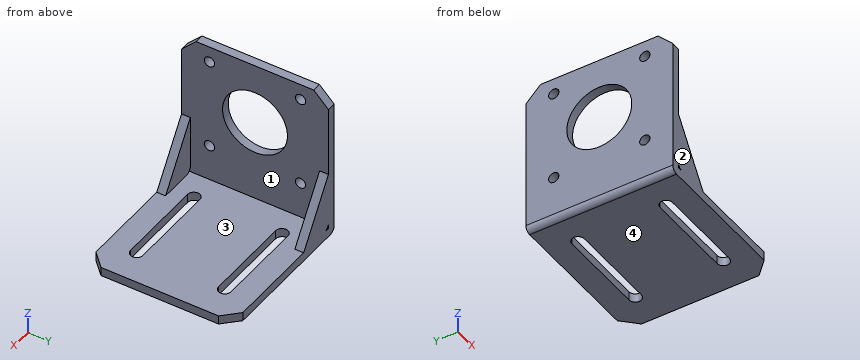
```python
from build123d import *

# Parameters (mm, degrees)
SKETCH_1_W      = 53
SKETCH_1_H      = 50
EXTRUDE_1_DEPTH = 3
SKETCH_2_W      = 49
SKETCH_2_H      = 50
SKETCH_2_R      = 11.05
SKETCH_2_R_2    = 1.75
EXTRUDE_2_DEPTH = 3
CHAMFER_1_SIZE  = 5
EXTRUDE_3_DEPTH = 3
FILLET_1_R      = 2


with BuildPart() as part:
    # 草图1 → 凸台-拉伸1 (new body)
    with BuildSketch(Plane.XY):
        Rectangle(SKETCH_1_W, SKETCH_1_H)
        with BuildLine():
            Line((-14.5, 17.103323548), (15.5, 17.103323548))
            ThreePointArc((15.5, 17.103323548), (17.603323548, 15), (15.5, 12.896676452))
            Line((15.5, 12.896676452), (-14.5, 12.896676452))
            ThreePointArc((-14.5, 12.896676452), (-16.603323548, 15), (-14.5, 17.103323548))
        make_face(mode=Mode.SUBTRACT)
        with BuildLine():
            Line((-14.5, -12.9), (15.5, -12.9))
            ThreePointArc((15.5, -12.9), (17.6, -15), (15.5, -17.1))
            Line((15.5, -17.1), (-14.5, -17.1))
            ThreePointArc((-14.5, -17.1), (-16.6, -15), (-14.5, -12.9))
        make_face(mode=Mode.SUBTRACT)
    extrude(amount=EXTRUDE_1_DEPTH)

    # 草图2 → 凸台-拉伸2 (add)
    with BuildSketch(Plane.ZY.offset(26.5)):
        with Locations((27.5, 0)):
            Rectangle(SKETCH_2_W, SKETCH_2_H)
        with Locations((31, 0)):
            Circle(SKETCH_2_R, mode=Mode.SUBTRACT)
        with Locations((46.5, 15.5)):
            Circle(SKETCH_2_R_2, mode=Mode.SUBTRACT)
        with Locations((46.5, -15.5)):
            Circle(SKETCH_2_R_2, mode=Mode.SUBTRACT)
        with Locations((15.5, -15.5)):
            Circle(SKETCH_2_R_2, mode=Mode.SUBTRACT)
        with Locations((15.5, 15.5)):
            Circle(SKETCH_2_R_2, mode=Mode.SUBTRACT)
    extrude(amount=-EXTRUDE_2_DEPTH)

    # 倒角1
    chamfer_1_edges = [part.edges().sort_by_distance(p)[0] for p in [
        (-25, 25, 52),
        (-25, -25, 52),
        (26.5, 25, 1.5),
        (26.5, -25, 1.5),
    ]]
    chamfer(chamfer_1_edges, length=CHAMFER_1_SIZE)

    # 草图3 → 凸台-拉伸3 (add)
    with BuildSketch(Plane.XZ.offset(25)):
        with BuildLine():
            Line((-23.5, 5), (-23.5, 23))
            Line((-23.5, 23), (-10.5, 3))
            Line((-10.5, 3), (-21.5, 3))
            ThreePointArc((-21.5, 3), (-22.914213562, 3.585786438), (-23.5, 5))
        make_face()
    extrude_3 = extrude(amount=-EXTRUDE_3_DEPTH)

    # 圆角1
    fillet_1_edges = [part.edges().sort_by_distance(p)[0] for p in [
        (-26.5, 0, 0),
    ]]
    fillet(fillet_1_edges, radius=FILLET_1_R)

    # 镜向1: 凸台-拉伸3 across plane
    add(extrude_3.mirror(Plane.ZX))


solid = part.part
```
Read the model definition and answer for the solid it produces. Units are mm, in the model's axes. Face numbers are marked on the shaded views. Give positions to 0.01 mm unless a question says otherwise; leave off trailing zeros. Write each loop counter-clockwise with the first axis right and the second up, starting at its lowest first coordinate (ties: lowest second). Pieces come first, ordered by that corner, then holes. Notation, with made-up numbers: (27.25, 69) -> (35.25, 69) arc R17 cw to (35.25, 81) -> close; hole circle Ø2 at (87, 29). An arc over 180 degrees is marked (long way). Answer as a JSON object with one key per item and string values.
1) Straight lines are drawn through the part: probe 1 along Y at (x, z) = (-24.8, 46.5); probe 2 along Y at (x, z) = (-24.75, 31); probe 3 along Z at (x, y) = (21, -21). For each, find the intervals that lie inside material, in ascending order. Write a range as from..to.
Findings below:
{"probe 1": "y = -25..-17.25, -13.75..13.75, 17.25..25", "probe 2": "y = -25..-11.05, 11.05..25", "probe 3": "z = 0..3"}
2) For a pull along Y with two mould halves and no side action, classify the marked faces 1, 2, 3 and 4 as pulls with the +Y half, pulls with the -Y half, needs draft (parallel to the pull), parting line crosses it, or undercut.
Findings below:
{"face 1": "undercut", "face 2": "pulls with the -Y half", "face 3": "undercut", "face 4": "needs draft"}
3) Section B-B on y = 0 is taken. Write down the section's boundary in (x, z).
Findings below:
{"outline": "(-26.5, 2) arc R2 ccw to (-24.5, 0) -> (26.5, 0) -> (26.5, 3) -> (-23.5, 3) -> (-23.5, 19.95) -> (-26.5, 19.95) -> close; (-26.5, 42.05) -> (-23.5, 42.05) -> (-23.5, 52) -> (-26.5, 52) -> close"}
4) Section D-D on y = 12 is taken. Write down the section's boundary in (x, z), then the cut area to 3 significant figures.
Findings below:
{"outline": "(-26.5, 2) arc R2 ccw to (-24.5, 0) -> (26.5, 0) -> (26.5, 3) -> (-23.5, 3) -> (-23.5, 52) -> (-26.5, 52) -> close", "area": "305 mm^2"}
5) Flat-ended cylindrical pins translate along their axes: pin 1 Ø5 at (y, z) = (-4.5, 16) entering from +X; pin 2 Ø2 at (y, z) = (15.5, 15.5) entering from -X; pin 3 Ø5 at (x, y) = (12, -4) entering from +Z. Find the tip coordinate at first contact, or state that the pin passes through.
Findings below:
{"pin 1": "stops at x = -23.5", "pin 2": "passes through", "pin 3": "stops at z = 3"}
6) Section C-C on z = 15.5 is taken. Write down the section's boundary in (x, y) (3 decimals), then the cut area to 3 significant figures.
Findings below:
{"outline": "(-26.5, -25) -> (-18.625, -25) -> (-18.625, -22) -> (-23.5, -22) -> (-23.5, -17.25) -> (-26.5, -17.25) -> close; (-26.5, -13.75) -> (-23.5, -13.75) -> (-23.5, 13.75) -> (-26.5, 13.75) -> close; (-26.5, 17.25) -> (-23.5, 17.25) -> (-23.5, 22) -> (-18.625, 22) -> (-18.625, 25) -> (-26.5, 25) -> close", "area": "158 mm^2"}
7) Section A-A on x = -0.5 is taken. Write down the section's boundary in (y, z).
Findings below:
{"outline": "(-25, 0) -> (-17.1, 0) -> (-17.1, 3) -> (-25, 3) -> close; (-12.9, 0) -> (12.9, 0) -> (12.9, 3) -> (-12.9, 3) -> close; (17.1, 0) -> (25, 0) -> (25, 3) -> (17.1, 3) -> close"}
